Can you work these out from the drawing? Everything is in mm from the part's minimum corner. A direction names the side the tool comes from. Coordinates: 2 decimals unless noted, no trailing zeros. Order: outer loops, then holes, each group sorted by start corner. A loop starts at its lowest first (then second) coordinate and runs counter-clockwise, first axis right, second up. Notation, with made-up numbers: M 19.5,74 L 41.5,74 A24 ccw 41.5,102 Z; hole C 3.25,-31 d7. An arc over 180 degrees is marked long. One line per question, with ' | ' between items. Start each with the question number.
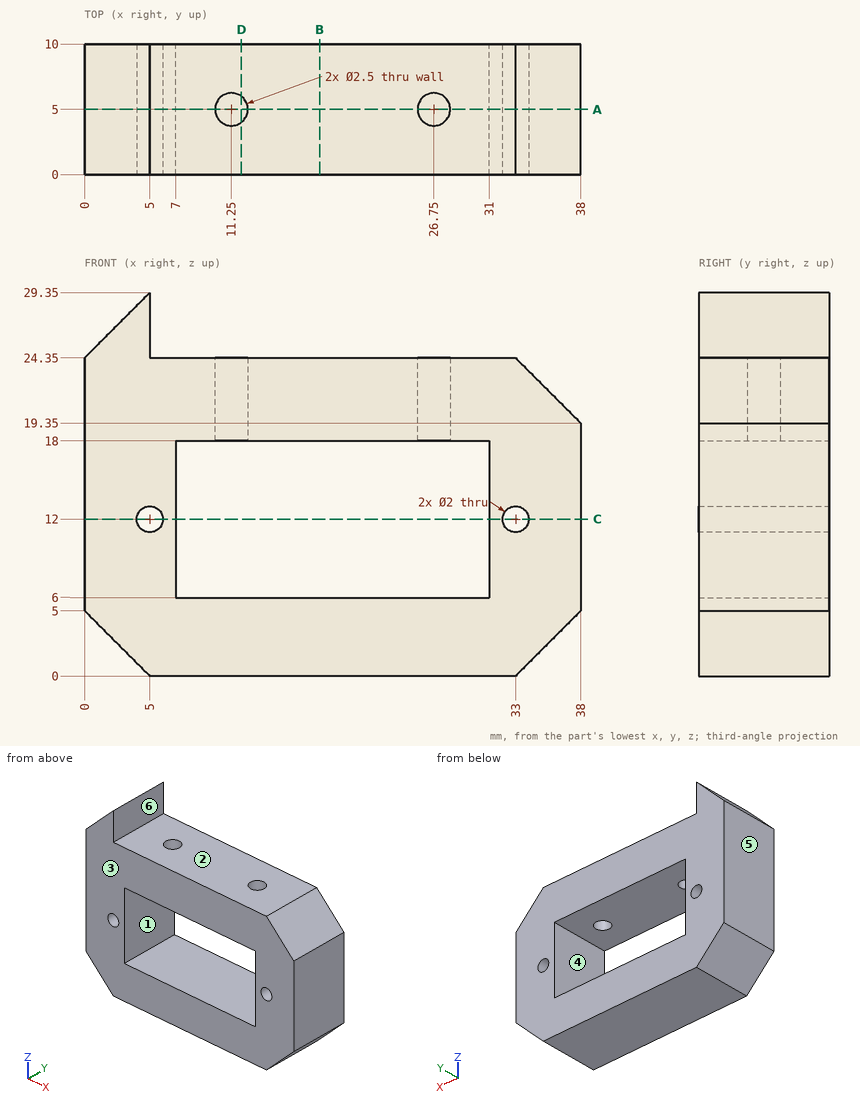
(1) Imagine slicing it at B-B, the plane x = 18. Write out the boundary of the cut face in (y, z), plus the area to 4 significant figures.
(2) Imagine slicing it at A-A, the plane y = 5. Count the separate pieces of the cut face and the enclosed holes in it, plus the area to 3 significant figures.
(3) If I drill on line 1 along X through (y, z) = (5.5, 12); line 2 along Z through (x, y) = (25.5, 9); line 3 along X through (y, z) = (1.5, 14.75), over which ranges is the centre line in solid material (lowest first)? Write a range as from..to.
(4) For P1, Ø3, axis at x = 33, z = 12, coming from the -Y side; P2, Ø2, axis at x = 26.75, y = 5, coming from the +Z side; P3, Ø1.2, axis at x = 5, z = 12, coming from the -Y side; P4, Ø2, axis at y = 3.5, z = 23.5, coming from the +X side, each with a flat end and sliding along its axis, tell me the tip position at first contact or that it passes through.
(5) On a 3-axis mill with a long thin cutter (end or side, diameter ignored), from which of +Z, -Z, +X, -X, +Y, -Y can I reach the whole of each face in a straight line? I mean the marked faces 4, 5 and 6. Say none if no direction works.
(6) Imagine slicing it at D-D, the plane x = 12. Write out the boundary of the cut face in (y, z).
(7) We'd pull the mould along Z, two halves only. Please class the marked faces 1, 2 and 3: +Z half, -Z half, draft (parallel to the pull), parting line (faces both ways), or undercut.
(8) Imagine slicing it at C-C, the plane z = 12. Write out the boundary of the cut face in (x, y).
Answers:
1) outline: M 0,0 L 10,0 L 10,6 L 0,6 Z; M 0,18 L 10,18 L 10,24.35 L 0,24.35 Z | area: 123.5 mm²
2) separate pieces: 2 | enclosed holes: 2 | area: 574 mm²
3) line 1: 0..4, 6..7, 31..32, 34..38 | line 2: 0..6, 18..24.35 | line 3: 0..7, 31..38
4) P1: y = 0 | P2: z = 6 | P3: through | P4: x = 34.85
5) face 4: +Y, -Y | face 5: +Z, -Z, -X, +Y, -Y | face 6: +Z, +X, +Y, -Y
6) outline: M 0,0 L 10,0 L 10,6 L 0,6 Z; M 0,18 L 4,18 L 4,24.35 L 0,24.35 Z; M 6,18 L 10,18 L 10,24.35 L 6,24.35 Z
7) face 1: undercut | face 2: +Z half | face 3: draft
8) outline: M 0,0 L 4,0 L 4,10 L 0,10 Z; M 6,0 L 7,0 L 7,10 L 6,10 Z; M 31,0 L 32,0 L 32,10 L 31,10 Z; M 34,0 L 38,0 L 38,10 L 34,10 Z
